The listing builds one solid part. Answer for the finished solid, in the listing's coordinates (mm). Give positions to 0.01 mm unless a question says otherwise; leave off trailing zeros. Order: outer loops, then holes, each group sorted by start corner. A loop starts at its lowest first (then second) coordinate and runs counter-clockwise, first axis right, second up. Notation, with made-up numbers: (-36, 45.5) - (-12, 45.5) arc R26 cw to (-12, 74.5) - close; hole circle Ø6 at (10, 68). An arc over 180 degrees is marked (long way). Answer in a Markdown table with one row per item.
from build123d import *

# Parameters (mm, degrees)
F0_R     = 60
F1_DEPTH = 4


with BuildPart() as f1:
    # F0 (on Top) → F1 (new body)
    with BuildSketch(Plane.XY):
        Circle(F0_R)
        with BuildLine():
            ThreePointArc((6, 46.184288), (7.316863, 48.662894), (10.106957, 48.967841))
            ThreePointArc((10.106957, 48.967841), (43.30127, 25), (47.460872, -15.731039))
            ThreePointArc((47.460872, -15.731039), (47.329687, -16.27085), (47.10122, -16.777219))
            ThreePointArc((47.10122, -16.777219), (45.281593, -18.189946), (42.996767, -17.895992))
            Line((42.996767, -17.895992), (16.13546, -6.450094))
            ThreePointArc((16.13546, -6.450094), (12.990381, -7.5), (13.653675, -10.748671))
            Line((13.653675, -10.748671), (36.996767, -28.288297))
            ThreePointArc((36.996767, -28.288297), (38.393752, -30.120037), (38.080108, -32.402244))
            ThreePointArc((38.080108, -32.402244), (37.755813, -32.853286), (37.353916, -33.236802))
            ThreePointArc((37.353916, -33.236802), (0, -50), (-37.353916, -33.236802))
            ThreePointArc((-37.353916, -33.236802), (-37.755813, -32.853286), (-38.080108, -32.402244))
            ThreePointArc((-38.080108, -32.402244), (-38.393752, -30.120037), (-36.996767, -28.288297))
            Line((-36.996767, -28.288297), (-13.653675, -10.748671))
            ThreePointArc((-13.653675, -10.748671), (-12.990381, -7.5), (-16.13546, -6.450094))
            Line((-16.13546, -6.450094), (-42.996767, -17.895992))
            ThreePointArc((-42.996767, -17.895992), (-45.281593, -18.189946), (-47.10122, -16.777219))
            ThreePointArc((-47.10122, -16.777219), (-47.329687, -16.27085), (-47.460872, -15.731039))
            ThreePointArc((-47.460872, -15.731039), (-43.30127, 25), (-10.106957, 48.967841))
            ThreePointArc((-10.106957, 48.967841), (-7.316863, 48.662894), (-6, 46.184288))
            Line((-6, 46.184288), (-2.481785, 17.198765))
            ThreePointArc((-2.481785, 17.198765), (0, 15), (2.481785, 17.198765))
            Line((2.481785, 17.198765), (6, 46.184288))
        make_face(mode=Mode.SUBTRACT)
    extrude(amount=F1_DEPTH)


solid = f1.part
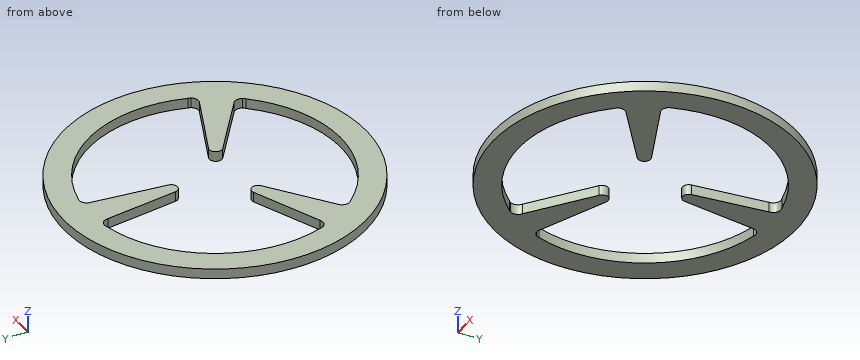
Item 1: Find section C-C on x = -21. Write down the section's boundary in (y, z), then the cut area to 3 significant figures.
Answer block:
| item | result |
|---|---|
| outline | (-56.2, 0) - (-45.38, 0) - (-45.38, 4) - (-56.2, 4) - close; (-16.27, 0) - (-8.52, 0) - (-8.52, 4) - (-16.27, 4) - close; (45.38, 0) - (56.2, 0) - (56.2, 4) - (45.38, 4) - close |
| area | 118 mm² |
Item 2: Find section A-A on x = 0. Write down the section's boundary in (y, z).
Answer block:
| item | result |
|---|---|
| outline | (-60, 0) - (-50, 0) - (-50, 4) - (-60, 4) - close; (15, 0) - (60, 0) - (60, 4) - (15, 4) - close |
Item 3: Consider line 1 (X direction, y = 1.5, z = 1.45); line 2 (Y direction, x = -38, z = 1.85); line 3 (Y direction, x = -24, z = 1.4). Determine where each line is inside the solid, lowest interval first.
Answer block:
| item | result |
|---|---|
| line 1 | -59.98 to -49.98, 49.98 to 59.98 |
| line 2 | -46.43 to -32.53, -29.24 to -15.77, 32.5 to 46.43 |
| line 3 | -54.99 to -43.86, -18.52 to -9.8, 43.86 to 54.99 |
Item 4: Each of these flat-tipped pins is pushed along its axis until it touches: P1, Ø6, axis at x = -28.5, y = -37.5, coming from the +Z side; P2, Ø1.5, axis at y = -13, z = 1.5, coming from the -X side; P3, Ø2, axis at x = 14.5, z = 1.5, coming from the -Y side; P4, Ø1.5, axis at y = 17.5, z = 3.5, coming from the -X side. Where does it stop, or does it pass through?
Answer block:
| item | result |
|---|---|
| P1 | z = 4 |
| P2 | x = -58.74 |
| P3 | y = -58.46 |
| P4 | x = -57.61 |
Item 5: Find section D-D on z = 3.2. Write down the section's boundary in (x, y), then the cut area to 3 significant figures.
Answer block:
| item | result |
|---|---|
| outline | circle Ø120 at (0, 0); hole (-47.46, -15.73) arc R3 ccw to (-47.1, -16.78) arc R3 ccw to (-43, -17.9) - (-16.14, -6.45) arc R2.5 cw to (-13.65, -10.75) - (-37, -28.29) arc R3 ccw to (-38.08, -32.4) arc R3 ccw to (-37.35, -33.24) arc R50 ccw to (37.35, -33.24) arc R3 ccw to (38.08, -32.4) arc R3 ccw to (37, -28.29) - (13.65, -10.75) arc R2.5 cw to (16.14, -6.45) - (43, -17.9) arc R3 ccw to (47.1, -16.78) arc R3 ccw to (47.46, -15.73) arc R50 ccw to (10.11, 48.97) arc R3 ccw to (6, 46.18) - (2.48, 17.2) arc R2.5 cw to (-2.48, 17.2) - (-6, 46.18) arc R3 ccw to (-10.11, 48.97) arc R50 ccw to start |
| area | 4,370 mm² |
Item 6: Find section B-B on y = 0. Write down the section's boundary in (x, z).
Answer block:
| item | result |
|---|---|
| outline | (-60, 0) - (-50, 0) - (-50, 4) - (-60, 4) - close; (50, 0) - (60, 0) - (60, 4) - (50, 4) - close |
